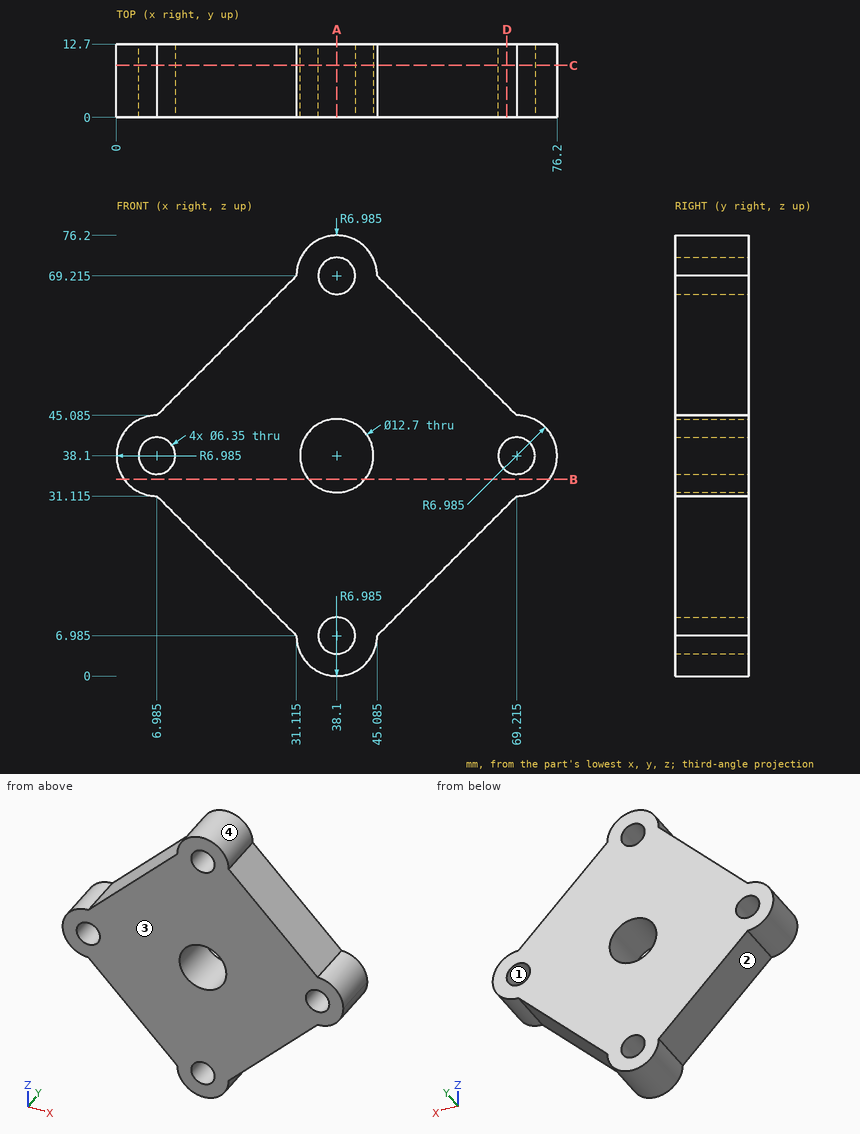
Check sheet for the drawn part. Datum: minimum x, y, z corner. Units: mm. Round coordinates to 2 decimals unless told otherwise and drop trailing zeros. Order: outer loops, then holes, each group sorted by start corner. A loop starts at its lowest first (then second) coordinate and runs counter-clockwise, first axis right, second up. Notation, with made-up numbers: M 23.25,78.5 L 50.25,78.5 A27 cw 50.25,103.5 Z; hole C 67,-12.5 d10. An arc over 180 degrees is marked long. Answer in a Markdown table with one row per item.
(1) Section check A-A on x = 38.1. Record the boundary of the cut face in (y, z), plus the area to 3 significant figures.
Findings:
| item | result |
|---|---|
| outline | M 0,0 L 12.7,0 L 12.7,3.81 L 0,3.81 Z; M 0,10.16 L 12.7,10.16 L 12.7,31.75 L 0,31.75 Z; M 0,44.45 L 12.7,44.45 L 12.7,66.04 L 0,66.04 Z; M 0,72.39 L 12.7,72.39 L 12.7,76.2 L 0,76.2 Z |
| area | 645 mm^2 |
(2) Draft check along Z on the marked faces 1, 2, 3 and 4. Enter one of: +Z half, -Z half, draft (parallel to the pull), parting line (faces both ways), or undercut.
Findings:
| item | result |
|---|---|
| face 1 | undercut |
| face 2 | -Z half |
| face 3 | draft |
| face 4 | +Z half |
(3) Material ranges on line 1 along Z through (x, y) = (38.1, 10.25); line 2 along X through (y, z) = (11, 38.5); line 3 along X through (y, z) = (5.5, 33.5), recorded low to high. Write a range as from..to.
Findings:
| item | result |
|---|---|
| line 1 | z = 0..3.81, 10.16..31.75, 44.45..66.04, 72.39..76.2 |
| line 2 | x = 0.01..3.84, 10.13..31.76, 44.44..66.07, 72.36..76.19 |
| line 3 | x = 1.73..33.72, 42.48..74.47 |
(4) Gauge pin test, flat ends, axial feed: pin 1 (6 mm diameter, centred on x = 27, y = 1.5, fed in from +Z); pin 2 (2 mm diameter, centred on x = 15.5, y = 7, fed in from -Z); pin 3 (5 mm diameter, centred on x = 53.5, y = 9.5, fed in from -Z). Record the tip position at first contact, or that the pin passes through.
Findings:
| item | result |
|---|---|
| pin 1 | stops at z = 68.1 |
| pin 2 | stops at z = 21.6 |
| pin 3 | stops at z = 12.9 |
(5) Section check B-B on z = 34. Record the boundary of the cut face in (x, y), plus the area to 3 significant figures.
Findings:
| item | result |
|---|---|
| outline | M 1.33,0 L 33.25,0 L 33.25,12.7 L 1.33,12.7 Z; M 42.95,0 L 74.87,0 L 74.87,12.7 L 42.95,12.7 Z |
| area | 811 mm^2 |
(6) Section check C-C on y = 9. Record the boundary of the cut face in (x, z) (3 decimals).
Findings:
| item | result |
|---|---|
| outline | M 6.985,31.115 L 31.115,6.985 A6.985 ccw 45.085,6.985 L 69.215,31.115 A6.985 ccw 69.215,45.085 L 45.085,69.215 A6.985 ccw 31.115,69.215 L 6.985,45.085 A6.985 ccw Z; hole C 6.985,38.1 d6.35; hole C 38.1,38.1 d12.7; hole C 38.1,6.985 d6.35; hole C 38.1,69.215 d6.35; hole C 69.215,38.1 d6.35 |
(7) Section check D-D on x = 67.5. Record the boundary of the cut face in (y, z).
Findings:
| item | result |
|---|---|
| outline | M 0,29.4 L 12.7,29.4 L 12.7,35.43 L 0,35.43 Z; M 0,40.77 L 12.7,40.77 L 12.7,46.8 L 0,46.8 Z |
